The model under review builds one solid part; all positions refer to its coordinate system, in mm. A direction names the side the tool comes from. Give positions to 0.01 mm unless a question says otherwise; leave off trailing zeros. Order: outer loops, then holes, each group sorted by start corner. A loop starts at its lowest first (then second) coordinate and runs counter-clockwise, first axis right, second up. Notation, with made-up numbers: (62.25, 5.5) - (72.25, 5.5) arc R21 ccw to (72.25, 39.5) - close; hole circle Ø1 at (19.5, 75.5). An arc over 180 degrees is marked (long way). Use CSV: the item, a comma, the result in double quotes. Start each with the question number.
1. For pin 1 (1.5 mm diameter, centred on x = 2, y = 4.5, fed in from +Z); pin 2 (1.6 mm diameter, centred on x = -51.5, z = 7.5, fed in from -Y); pin 3 (3 mm diameter, centred on y = 4.5, z = 5, fed in from +X), all flat-tipped, find the tip position at first contact; note any pin that passes through.
2. Take a section at D-D, the plane y = -12. State the section outline as (x, z) points, then the cut area to 4 significant figures.
3. Machinability: for faces 1 (the flat face through (68.37, -4, 9)), 2 (the flat face through (73.279, 5, 1)), which of the approach directions +Z, -Z, +X, -X, +Y, -Y give a long, thin tool a straight path to every point of the face, cutting with its end or side? Answer none if there is none.
4. To check wall thickness, follow line 1 (X direction, y = -19, z = 5); line 2 (Y direction, x = -20, z = 9.5); line 3 (Z direction, x = 21.5, y = 21). State the ranges of each line that lie inside material, in increasing order. Write a range as [from, to].
5. Draft analysis for pull direction X (two halves, no side actions). For faces 3 (the flat face through (-52.221, 5, 8)), 4 (the cylindrical face through (60.786, 31.605, 1.993)), 5 (the flat face through (10, -23.36, 8)), state which applies: released by +X, released by -X, zero draft, split by the parting line, or undercut.
6. Take a section at B-B, the plane y = 15. State the section outline as (x, z) points.
7. Take a section at A-A, the plane x = -21. State the section outline as (y, z) points.
8. Take a section at C-C, the plane z = 9. Count the separate pieces of the cut face and the enclosed holes in it, then the cut area to 3 significant figures.
```python
from build123d import *

# Parameters (mm, degrees)
F0_W      = 125.5
F0_H      = 58
F1_DEPTH  = 15.5
F2_W      = 122.5
F2_H      = 55
F3_DEPTH  = 14
F4_W      = 1.5
F4_H      = 13
F4_H_2    = 10
F5_DEPTH  = 12.5
F6_R      = 1.5
F7_DEPTH  = 2
F8_R      = 1
F9_R      = 2
F10_R     = 2
F11_W     = 1.5
F11_H     = 19
F12_DEPTH = 14
F13_W     = 1.1
F13_H     = 2.109523
F13_W_2   = 1.309524
F13_H_2   = 2.976188
F14_DEPTH = 14


with BuildPart() as f1:
    # F0 (on Top) → F1 (new body)
    with BuildSketch(Plane.XY):
        with Locations((10.529152, 5.640338)):
            Rectangle(F0_W, F0_H)
    extrude(amount=F1_DEPTH)

    # F2 (on face) → F3 (cut)
    with BuildSketch(Plane.XY.offset(15.5)):
        with Locations((10.529152, 5.640338)):
            Rectangle(F2_W, F2_H)
    extrude(amount=-F3_DEPTH, mode=Mode.SUBTRACT)

    # F4 (on face) → F5 (cut)
    with BuildSketch(Plane.XY.offset(15.5)):
        with Locations((-51.470848, 16.640338)):
            Rectangle(F4_W, F4_H)
        with Locations((-51.470848, -12.609662)):
            Rectangle(F4_W, F4_H_2)
    extrude(amount=-F5_DEPTH, mode=Mode.SUBTRACT)

    # F6 (on face) → F7 (join)
    with BuildSketch(Plane.XY.offset(1.5)):
        with Locations((-35.220848, 30.340338)):
            Circle(F6_R)
        with Locations((59.979152, 30.340338)):
            Circle(F6_R)
        with Locations((66.779152, -19.059662)):
            Circle(F6_R)
        with Locations((-36.220848, -19.059662)):
            Circle(F6_R)
    extrude(amount=F7_DEPTH)

    # F8
    f8_edges = [f1.edges().sort_by_distance(p)[0] for p in [
        (-36.720848, 30.340338, 3.5),
        (58.479152, 30.340338, 3.5),
        (-37.720848, -19.059662, 3.5),
        (65.279152, -19.059662, 3.5),
    ]]
    fillet(f8_edges, radius=F8_R)

    # F9
    f9_edges = [f1.edges().sort_by_distance(p)[0] for p in [
        (-52.220848, 34.640338, 7.75),
        (-52.220848, -23.359662, 7.75),
        (73.279152, -23.359662, 7.75),
        (73.279152, 34.640338, 7.75),
    ]]
    fillet(f9_edges, radius=F9_R)

    # F10
    f10_edges = [f1.edges().sort_by_distance(p)[0] for p in [
        (-50.720848, 33.140338, 8.5),
        (71.779152, -21.859662, 8.5),
        (71.779152, 33.140338, 8.5),
        (-50.720848, -21.859662, 8.5),
    ]]
    fillet(f10_edges, radius=F10_R)

    # F11 (on face) → F12 (cut)
    with BuildSketch(Plane.XY.offset(15.5)):
        with Locations((72.529152, 7.359652)):
            Rectangle(F11_W, F11_H)
    extrude(amount=-F12_DEPTH, mode=Mode.SUBTRACT)

    # F13 (on face) → F14 (join)
    with BuildSketch(Plane.XY.offset(15.5)):
        with Locations((69.129152, 17.914414)):
            Rectangle(F13_W, F13_H)
        with Locations((69.02439, -3.628442)):
            Rectangle(F13_W_2, F13_H_2)
    extrude(amount=-F14_DEPTH)


solid = f1.part
```
Determined:
1,pin 1,"stops at z = 1.5"
1,pin 2,"stops at y = -23.3"
1,pin 3,"stops at x = -50.72"
2,outline,"(-52.22, 0) - (73.28, 0) - (73.28, 15.5) - (71.78, 15.5) - (71.78, 1.5) - (-50.72, 1.5) - (-50.72, 3) - (-52.22, 3) - close"
2,area,"211.5 mm²"
3,face 1,"+Z"
3,face 2,"+Z, -Z, +X, +Y, -Y"
4,line 1,"x = [-52.22, -50.72], [71.78, 73.28]"
4,line 2,"y = [-23.36, -21.86], [33.14, 34.64]"
4,line 3,"z = [0, 1.5]"
5,face 3,"released by -X"
5,face 4,"undercut"
5,face 5,"zero draft"
6,outline,"(-52.22, 0) - (73.28, 0) - (73.28, 1.5) - (-50.72, 1.5) - (-50.72, 3) - (-52.22, 3) - close"
7,outline,"(-23.36, 0) - (34.64, 0) - (34.64, 15.5) - (33.14, 15.5) - (33.14, 1.5) - (-21.86, 1.5) - (-21.86, 15.5) - (-23.36, 15.5) - close"
8,separate pieces,"5"
8,enclosed holes,"0"
8,area,"485 mm²"
